from build123d import *

# Parameters (mm, degrees)
SKETCH_1_R      = 45
SKETCH_1_R_2    = 2
EXTRUDE_1_DEPTH = 5
SKETCH_2_R      = 47
SKETCH_2_R_2    = 45
EXTRUDE_2_DEPTH = 68.18


with BuildPart() as part:
    # 草图1 → 凸台-拉伸1 (new body)
    with BuildSketch(Plane(origin=(0, 0, 0), x_dir=(1, 0, 0), z_dir=(0, 1, 0))):
        with BuildLine():
            Line((50.697633081, 20), (80.5, 20))
            Line((80.5, 20), (80.5, -20))
            Line((80.5, -20), (50.697633081, -20))
            ThreePointArc((50.697633081, -20), (0, -54.5), (-50.697633081, -20))
            Line((-50.697633081, -20), (-80.5, -20))
            Line((-80.5, -20), (-80.5, 20))
            Line((-80.5, 20), (-50.697633081, 20))
            ThreePointArc((-50.697633081, 20), (0, 54.5), (50.697633081, 20))
        make_face()
        Circle(SKETCH_1_R, mode=Mode.SUBTRACT)
        with Locations((76, -14.8)):
            Circle(SKETCH_1_R_2, mode=Mode.SUBTRACT)
        with Locations((61, -14.8)):
            Circle(SKETCH_1_R_2, mode=Mode.SUBTRACT)
        with Locations((76, 14.8)):
            Circle(SKETCH_1_R_2, mode=Mode.SUBTRACT)
        with Locations((61, 14.8)):
            Circle(SKETCH_1_R_2, mode=Mode.SUBTRACT)
        with Locations((-61, 14.8)):
            Circle(SKETCH_1_R_2, mode=Mode.SUBTRACT)
        with Locations((-76, 14.8)):
            Circle(SKETCH_1_R_2, mode=Mode.SUBTRACT)
        with Locations((-76, -14.8)):
            Circle(SKETCH_1_R_2, mode=Mode.SUBTRACT)
        with Locations((-61, -14.8)):
            Circle(SKETCH_1_R_2, mode=Mode.SUBTRACT)
    extrude(amount=EXTRUDE_1_DEPTH)

    # 草图2 → 凸台-拉伸2 (add)
    with BuildSketch(Plane(origin=(0, 5, 0), x_dir=(1, 0, 0), z_dir=(0, 1, 0))):
        Circle(SKETCH_2_R)
        Circle(SKETCH_2_R_2, mode=Mode.SUBTRACT)
    extrude(amount=EXTRUDE_2_DEPTH)


solid = part.part
Build history of the part. All positions in model axes, mm. A direction names the side the tool comes from. Round coordinates to 2 decimals unless told otherwise and drop trailing zeros. Write each loop counter-clockwise with the first axis right and the second up, starting at its lowest first coordinate (ties: lowest second). Pieces come first, ordered by that corner, then holes. Notation, with made-up numbers: (63.5, 88) - (97.5, 88) arc R23 cw to (97.5, 99) - close; hole circle Ø2 at (62, 87). An arc over 180 degrees is marked (long way). Use CSV: the item, a comma, the result in double quotes.
(1) Band-saw the part on D-D (y = 10). Write the cut outline in (x, z).
Response:
outline,"circle Ø94 at (0, 0); hole circle Ø90 at (0, 0)"
(2) Band-saw the part on A-A (x = 0). Write the cut outline in (y, z), plus the area to 3 significant figures.
Response:
outline,"(0, -54.5) - (5, -54.5) - (5, -47) - (73.18, -47) - (73.18, -45) - (0, -45) - close; (0, 45) - (73.18, 45) - (73.18, 47) - (5, 47) - (5, 54.5) - (0, 54.5) - close"
area,"368 mm²"
(3) Band-saw the part on C-C (x = -76). Write the cut outline in (y, z).
Response:
outline,"(0, -20) - (5, -20) - (5, -16.8) - (0, -16.8) - close; (0, -12.8) - (5, -12.8) - (5, 12.8) - (0, 12.8) - close; (0, 16.8) - (5, 16.8) - (5, 20) - (0, 20) - close"
(4) Band-saw the part on B-B (z = 0). Write the cut outline in (x, y), plus the area to 3 significant figures.
Response:
outline,"(-80.5, 0) - (-45, 0) - (-45, 73.18) - (-47, 73.18) - (-47, 5) - (-80.5, 5) - close; (45, 0) - (80.5, 0) - (80.5, 5) - (47, 5) - (47, 73.18) - (45, 73.18) - close"
area,"628 mm²"
(5) Wall check: line 1 (Z direction, x = -61, y = 1.65); line 2 (X direction, y = 3.1, z = 14.8); line 3 (X direction, y = 68, z = 1). Give the ranges that are in metal, low to high.
Response:
line 1,"-20 to -16.8, -12.8 to 12.8, 16.8 to 20"
line 2,"-80.5 to -78, -74 to -63, -59 to -42.5, 42.5 to 59, 63 to 74, 78 to 80.5"
line 3,"-46.99 to -44.99, 44.99 to 46.99"
(6) 3-axis set-ups, long thin cutter, end or side, ignore diameter. For faces 1 (the flat face through (-65, 2, 20)), 2 (the cylindrical face through (44.83, 38.61, -14.12)), 3 (the flat face through (-66, 2, -20)): which of +Z, -Z, +X, -X, +Y, -Y reach the whole face in a straight line?
Response:
face 1,"+Z, -X, +Y, -Y"
face 2,"+Y"
face 3,"-Z, -X, +Y, -Y"
(7) Mould opens along X. For faces 4 (the flat face through (80.5, 2, 0)), 5 (the flat face through (-80.5, 2, 0)), 6 (the cylindrical face through (60.566, 2.465, -12.848)) say: pulls with the +X half, pulls with the -X half, needs draft (parallel to the pull), parting line crosses it, or undercut.
Response:
face 4,"pulls with the +X half"
face 5,"pulls with the -X half"
face 6,"undercut"
(8) Pin check, flat tips, straight feed: P1, Ø4, axis at x = 31, y = 10.5, coming from the +Z side; P2, Ø4.5, axis at x = 61, z = -14.8, coming from the -Y side; P3, Ø3, axis at x = 40, z = 13.5, coming from the -Y side (3 decimals); P4, Ø4, axis at x = 12, y = 62, coming from the +Z side. Stop position of each tip, or through.
Response:
P1,"z = 36.99"
P2,"y = 0"
P3,"through"
P4,"z = 45.92"
